```python
from build123d import *

# Parameters (mm, degrees)
SKETCH1_R            = 30
BOSS_EXTRUDE1_DEPTH  = 3
SKETCH2_W            = 7
SKETCH2_H            = 50
BOSS_EXTRUDE2_DEPTH  = 2
SKETCH3_R            = 30
BOSS_EXTRUDE3_DEPTH  = 3
SKETCH4_W            = 7
SKETCH4_H            = 50
BOSS_EXTRUDE4_DEPTH  = 2
SKETCH5_R            = 30
BOSS_EXTRUDE5_DEPTH  = 3
SKETCH6_W            = 7
SKETCH6_H            = 50
BOSS_EXTRUDE6_DEPTH  = 2
SKETCH7_R            = 30
BOSS_EXTRUDE7_DEPTH  = 30
SKETCH8_R            = 27
CUT_EXTRUDE3_DEPTH   = 27
CUT_EXTRUDE6_START   = -15
CUT_EXTRUDE6_DEPTH   = 15
BOSS_EXTRUDE11_START = -30.000001
SKETCH14_R           = 5
BOSS_EXTRUDE11_DEPTH = 60.000002


with BuildPart() as part:
    # Sketch1 → Boss-Extrude1 (new body)
    with BuildSketch(Plane(origin=(0, 0, 0), x_dir=(0, 0, -1), z_dir=(1, 0, 0))):
        Circle(SKETCH1_R)
    extrude(amount=BOSS_EXTRUDE1_DEPTH)

    # Sketch2 → Boss-Extrude2 (add)
    with BuildSketch(Plane(origin=(3, 0, 0), x_dir=(0, 0, -1), z_dir=(1, 0, 0))):
        Rectangle(SKETCH2_W, SKETCH2_H)
    extrude(amount=BOSS_EXTRUDE2_DEPTH)

    # Sketch3 → Boss-Extrude3 (add)
    with BuildSketch(Plane(origin=(5, 0, 0), x_dir=(0, 0, -1), z_dir=(1, 0, 0))):
        Circle(SKETCH3_R)
    extrude(amount=BOSS_EXTRUDE3_DEPTH)

    # Sketch4 → Boss-Extrude4 (add)
    with BuildSketch(Plane(origin=(8, 0, 0), x_dir=(0, 0, -1), z_dir=(1, 0, 0))):
        Rectangle(SKETCH4_W, SKETCH4_H)
    extrude(amount=BOSS_EXTRUDE4_DEPTH)

    # Sketch5 → Boss-Extrude5 (add)
    with BuildSketch(Plane(origin=(10, 0, 0), x_dir=(0, 0, -1), z_dir=(1, 0, 0))):
        Circle(SKETCH5_R)
    extrude(amount=BOSS_EXTRUDE5_DEPTH)

    # Sketch6 → Boss-Extrude6 (add)
    with BuildSketch(Plane(origin=(13, 0, 0), x_dir=(0, 0, -1), z_dir=(1, 0, 0))):
        Rectangle(SKETCH6_W, SKETCH6_H)
    extrude(amount=BOSS_EXTRUDE6_DEPTH)

    # Sketch7 → Boss-Extrude7 (add)
    with BuildSketch(Plane(origin=(15, 0, 0), x_dir=(0, 0, -1), z_dir=(1, 0, 0))):
        Circle(SKETCH7_R)
    extrude(amount=BOSS_EXTRUDE7_DEPTH)

    # Sketch8 → Cut-Extrude3 (cut)
    with BuildSketch(Plane(origin=(45, 0, 0), x_dir=(0, 0, -1), z_dir=(1, 0, 0))):
        Circle(SKETCH8_R)
    extrude(amount=-CUT_EXTRUDE3_DEPTH, mode=Mode.SUBTRACT)

    # Sketch9 → Cut-Extrude6 (cut)
    with BuildSketch(Plane(origin=(45, 0, 0), x_dir=(0, 0, -1), z_dir=(1, 0, 0)).offset(CUT_EXTRUDE6_START)):
        with BuildLine():
            Line((21.213203436, 21.213203436), (19.091883092, 19.091883092))
            ThreePointArc((19.091883092, 19.091883092), (27, 0), (19.091883092, -19.091883092))
            Line((19.091883092, -19.091883092), (21.213203436, -21.213203436))
            ThreePointArc((21.213203436, -21.213203436), (30, 0), (21.213203436, 21.213203436))
        make_face()
        with BuildLine():
            Line((-21.213203436, 21.213203436), (-19.091883092, 19.091883092))
            ThreePointArc((-19.091883092, 19.091883092), (-27, 0), (-19.091883092, -19.091883092))
            Line((-19.091883092, -19.091883092), (-21.213203436, -21.213203436))
            ThreePointArc((-21.213203436, -21.213203436), (-30, 0), (-21.213203436, 21.213203436))
        make_face()
    extrude(amount=CUT_EXTRUDE6_DEPTH, mode=Mode.SUBTRACT)

    # Sketch14 → Boss-Extrude11 (add)
    with BuildSketch(Plane(origin=(0, 0, 0), x_dir=(1, 0, 0), z_dir=(0, 1, 0)).offset(BOSS_EXTRUDE11_START)):
        with Locations(Location((37.056780036, 0, 0), (0, 0, 90))):
            Circle(SKETCH14_R)
    extrude(amount=BOSS_EXTRUDE11_DEPTH)


solid = part.part
```
Geometry: final body of the model. Coordinates: model frame, mm. A direction names the side the tool comes from. Round coordinates to 2 decimals unless told otherwise and drop trailing zeros. Loops run counter-clockwise (first coordinate to the right, second up) from the corner with the lowest first, then second, coordinate; pieces in that order, holes last. Notation, with made-up numbers: (14, -12) -> (45, -12) arc R23 ccw to (45, 22) -> close; hole circle Ø9 at (11.5, -34.75). An arc over 180 degrees is marked (long way). Use one line per item in the form item = value. Start each with the question number.
1) Draft query along X for faces 5 (the flat face through (9, 25, 0)), 6 (the flat face through (0, 0, 0)), 7 (the flat face through (30, 0.1, 27.3)). Return one class per face: released by +X, released by -X, zero draft, split by the parting line, or undercut.
2) Section B-B on x = 19. Output: boundary loops of the cut face in (y, z), then the cut area to 3 significant figures.
3) First-contact query: P1, Ø0.6, axis at x = 4.5, y = 8, coming from the -Z side; P2, Ø0.6, axis at x = 14.5, y = -3.5, coming from the +Z side; P3, Ø5.5, axis at y = -8.5, z = -23.5, coming from the +X side. Flat tips, straight axial feed; report the tip coordinate or a pass-through.
4) Line query: L1, parallel to X at y = 2, z = -17; L2, parallel to Z at x = 28, y = 0. Output: solid intervals per line, ascending.
5) Access query for faces 1 (the flat face through (4, 0, -3.5)), 2 (the cylindrical face through (40.099, -0.378, 3.968)), 3 (the flat face through (14, 0, 3.5)), 4 (the flat face through (14, -25, 0)). Directions: +Z, -Z, +X, -X, +Y, -Y. A direction counts if a zero-diameter tool reaches every point of the face in a straight line with its end or side. Return the directions, or none.
Response:
q1.face_5 = undercut
q1.face_6 = released by -X
q1.face_7 = released by +X
q2.outline = circle Ø60 at (0, 0); hole circle Ø54 at (0, 0)
q2.area = 537 mm^2
q3.P1 = -3.5
q3.P2 = 3.5
q3.P3 = 30
q4.L1 = 0 to 3, 5 to 8, 10 to 13, 15 to 18
q4.L2 = -30 to -27, 27 to 30
q5.face_1 = -Z, +Y, -Y
q5.face_2 = none
q5.face_3 = +Z, +Y, -Y
q5.face_4 = +Z, -Z, -Y
